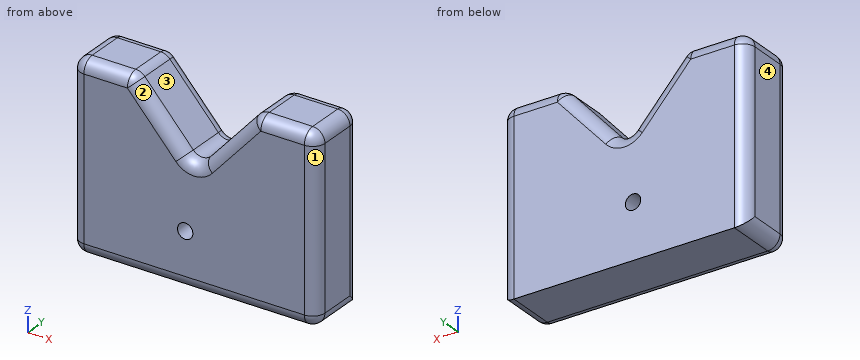
```python
from build123d import *

# Parameters (mm, degrees)
F1_DEPTH = 25.4
F2_R     = 5.08
F4_D     = 6.35


with BuildPart() as f1:
    # F0 (on Front) → F1 (new body)
    with BuildSketch(Plane.XZ):
        Polygon((-47.108385, 8.83777), (-47.108385, -67.36223), (54.491615, -67.36223), (54.491615, 8.83777), (29.091615, 8.83777), (3.691615, -19.560294), (-21.708385, 8.83777), align=None)
    extrude(amount=F1_DEPTH)

    # F2
    f2_edges = [f1.edges().sort_by_distance(p)[0] for p in [
        (-21.708385, -12.7, 8.83777),
        (-47.108385, -12.7, 8.83777),
        (-34.408385, 0, 8.83777),
        (-34.408385, -25.4, 8.83777),
        (54.491615, -12.7, 8.83777),
        (29.091615, -12.7, 8.83777),
        (41.791615, 0, 8.83777),
        (41.791615, -25.4, 8.83777),
        (54.491615, -12.7, -67.36223),
        (54.491615, 0, -29.26223),
        (54.491615, -25.4, -29.26223),
        (-47.108385, -25.4, -29.26223),
        (3.691615, -25.4, -67.36223),
        (16.391615, -25.4, -5.361262),
        (-9.008385, -25.4, -5.361262),
        (3.691615, -12.7, -19.560294),
        (-9.008385, 0, -5.361262),
        (16.391615, 0, -5.361262),
        (-47.108385, -12.7, -67.36223),
        (-47.108385, 0, -29.26223),
    ]]
    fillet(f2_edges, radius=F2_R)

    # F4 (through all)
    with Locations(Plane.XZ.offset(25.4)):
        with Locations((0, -44.623341)):
            Hole(F4_D / 2)


solid = f1.part
```
Verification items for the finished model (mm, model axes). Face numbers are marked on the shaded views. Coordinates: 2 decimals unless noted, no trailing zeros. Order: outer loops, then holes, each group sorted by start corner. A loop starts at its lowest first (then second) coordinate and runs counter-clockwise, first axis right, second up. Notation, with made-up numbers: (48, 2.5) - (78, 2.5) arc R7 ccw to (78, 6.5) - close; hole circle Ø5 at (1.5, 87.5). An arc over 180 degrees is marked (long way). Return JSON: item names as keys, results as strings.
(1) Mould release check, pull along X, two halves, no side actions. Record for the marked faces 1, 2, 3 and 4: pulls with the +X half, pulls with the -X half, needs draft (parallel to the pull), parting line crosses it, or undercut.
Filled sheet:
{"face 1": "pulls with the +X half", "face 2": "undercut", "face 3": "undercut", "face 4": "pulls with the -X half"}
(2) Section check B-B, the plane y = -4. Record the cut outline in (x, z) (3 decimals).
Filled sheet:
{"outline": "(-46.992, -63.362) arc R5.08 ccw to (-42.028, -67.362) - (49.412, -67.362) arc R5.08 ccw to (54.375, -63.362) - (54.375, 3.758) arc R4.964 ccw to (49.412, 8.722) - (31.363, 8.722) arc R4.964 ccw to (27.664, 7.067) - (7.565, -15.404) arc R5.196 cw to (-0.181, -15.404) - (-20.28, 7.067) arc R4.964 ccw to (-23.98, 8.722) - (-42.028, 8.722) arc R4.964 ccw to (-46.992, 3.758) - close; hole circle Ø6.35 at (0, -44.623)"}
(3) Go/stop test with flat-tipped pins: pin 1 (2 mm diameter, centred on y = -21.5, z = -49, fed in from -X); pin 2 (5 mm diameter, centred on x = 20, y = -10.5, fed in from +Z); pin 3 (6 mm diameter, centred on x = 1.5, y = -8.5, fed in from +Z). Record where each tip stops, or that it passes through.
Filled sheet:
{"pin 1": "stops at x = -47.11", "pin 2": "stops at z = 1.47", "pin 3": "stops at z = -13.76"}
(4) Thickness scan on line 1 along Z through (x, y) = (0, -10); line 2 along X through (y, z) = (-1.5, -12); line 3 along X through (y, z) = (-22.5, -2.5). Record the ranges inside material, lowest first.
Filled sheet:
{"line 1": "z = -67.36 to -47.8, -41.45 to -15.43", "line 2": "x = -45.63 to -5.05, 12.43 to 53.02", "line 3": "x = -46.62 to -12.23, 19.61 to 54"}
(5) Section check A-A, the plane y = -23. Record the cut outline in (x, z) (3 decimals).
Filled sheet:
{"outline": "(-46.344, -62.282) arc R4.316 ccw to (-42.028, -66.598) - (49.412, -66.598) arc R4.316 ccw to (53.727, -62.282) - (53.727, 3.758) arc R4.316 ccw to (49.412, 8.073) - (31.363, 8.073) arc R4.316 ccw to (28.147, 6.635) - (8.048, -15.837) arc R5.844 cw to (-0.665, -15.837) - (-20.764, 6.635) arc R4.316 ccw to (-23.98, 8.073) - (-42.028, 8.073) arc R4.316 ccw to (-46.344, 3.758) - close; hole circle Ø6.35 at (0, -44.623)"}
